Verification items for this drawing (mm, ordinates from the low corner). Coordinates: 2 decimals unless noted, no trailing zeros. Order: outer loops, then holes, each group sorted by start corner. A loop starts at its lowest first (then second) coordinate and runs counter-clockwise, first axis right, second up. Notation, with made-up numbers: M 19.25,49 L 62.25,49 A19 ccw 62.25,62 Z; hole C 73.5,-36 d3. An arc over 180 degrees is marked long. Return JSON: item names as keys, results as strings. Group by question number.
1. Section check A-A, the plane x = 8. Record the cut outline in (y, z).
2. Material ranges on line 1 along X through (y, z) = (73.5, 4.65); line 2 along Y through (x, z) = (6, 2.3); line 3 along Y through (x, z) = (40.5, 2.75), recorded low to high.
3. Section check B-B, the plane z = 1.1. Record the cut outline in (x, y) (1 decimal).
4. Section check D-D, the plane x = 56.5. Record the cut outline in (y, z).
5. Gauge pin test, flat ends, axial feed: pin 1 (1 mm diameter, centred on x = 17.5, z = 4, fed in from -Y); pin 2 (1.5 mm diameter, centred on y = 90.5, z = 1.5, fed in from +X); pin 3 (3 mm diameter, centred on y = 78.5, z = 3.5, fed in from -X). Record the tip position at first contact, or that the pin passes through.
6. Section check C-C, the plane y = 17. Record the cut outline in (x, z), plus the area to 3 significant figures.
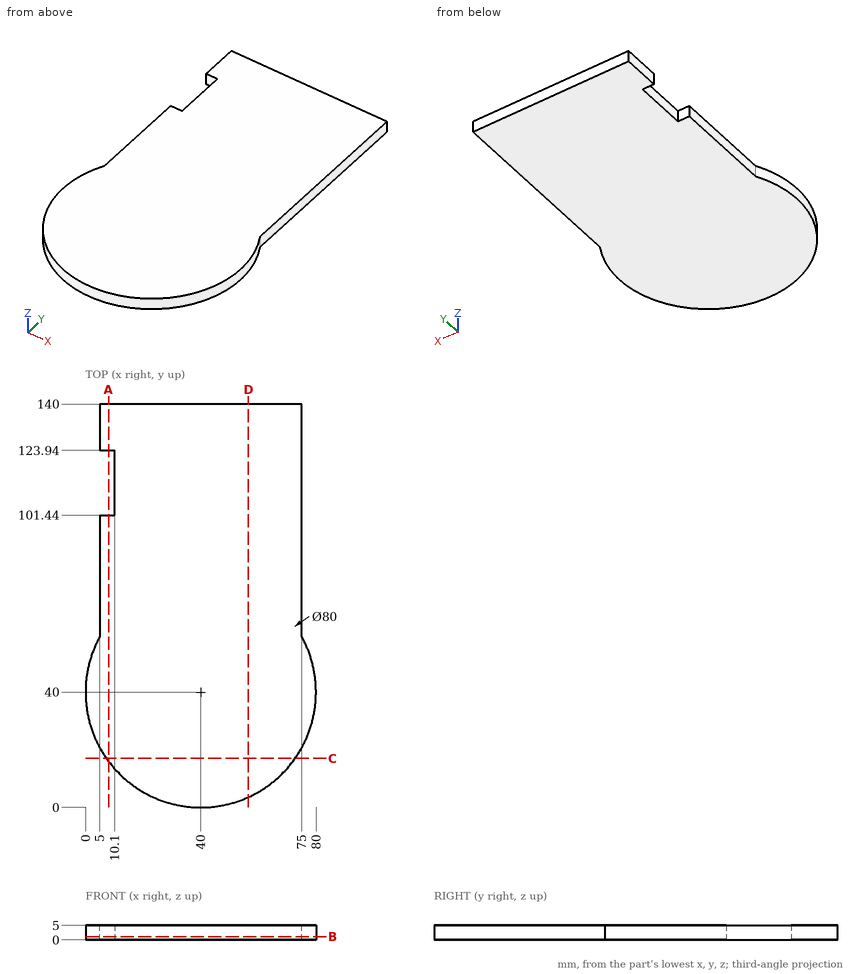
Answers follow:
{
 "1": {"outline": "M 16,0 L 101.44,0 L 101.44,5 L 16,5 Z; M 123.94,0 L 140,0 L 140,5 L 123.94,5 Z"},
 "2": {"line 1": "5 to 75", "line 2": "18.93 to 101.44, 123.94 to 140", "line 3": "0 to 140"},
 "3": {"outline": "M 5,59.4 A40 ccw long 75,59.4 L 75,140 L 5,140 L 5,123.9 L 10.1,123.9 L 10.1,101.4 L 5,101.4 Z"},
 "4": {"outline": "M 3.56,0 L 140,0 L 140,5 L 3.56,5 Z"},
 "5": {"pin 1": "y = 6.59", "pin 2": "x = 75", "pin 3": "x = 5"},
 "6": {"outline": "M 7.27,0 L 72.73,0 L 72.73,5 L 7.27,5 Z", "area": "327 mm^2"}
}
